Autodesk Inventor part; units mm, degrees
ref_plane "YZ Plane" through (0, 0, 0) normal (1, 0, 0) x (0, 1, 0)
ref_plane "XZ Plane" through (0, 0, 0) normal (0, 1, 0) x (-1, 0, 0)
ref_plane "XY Plane" through (0, 0, 0) normal (0, 0, 1) x (1, 0, 0)
ref_plane "Work Plane1" through (-71.5431, 15.4261, 39.8011) normal (1, 0, 0) x (0, -1, 0)
sketch "Sketch1" plane through (-71.5431, 15.4261, 39.8011) normal (1, 0, 0) x (0, -1, 0)
  circle A0 centre (-40.9, -21) radius 3
  circle A1 centre (-1.5, -21) radius 3
  line L0 (-45.9, -13) -> (3.5, -13)
  line L1 (3.5, -13) -> (3.5, -35)
  line L2 (3.5, -35) -> (-45.9, -35)
  line L3 (-45.9, -35) -> (-45.9, -13)
  line L4 (66.8457, -32) -> (-83.1543, -32)
  point P0 (15.4261, 39.8011)
  dimension "d0" = 5
  dimension "d1" = 8
  dimension "d2" = 5
  dimension "d3" = 3
extrude "Extrusion1" add sketch "Sketch1" along normal blind 12
sketch "Sketch2" plane through (-71.5431, 11.9261, 52.8011) normal (0, -1, 0) x (1, 0, 0)
  circle A0 centre (8.688, 16) radius 3
  circle A1 centre (8.688, 16) radius 3.75
  point P0 (71.5431, -52.8011)
  dimension "d6" = 7.5
extrude "Extrusion2" cut sketch "Sketch2" against normal through all contours A0 | A1
ref_plane "Work Plane2" through (-71.5431, 36.6261, 52.8011) normal (0, -1, 0) x (1, 0, 0)
sketch "Sketch3" plane through (-71.5431, 36.6261, 52.8011) normal (0, -1, 0) x (1, 0, 0)
  circle A0 centre (8.688, 16) radius 6
  circle A1 centre (8.688, 16) radius 6.5
  point P0 (71.5431, -52.8011)
  dimension "d9" = 0.5
extrude "Extrusion3" cut sketch "Sketch3" along normal mid plane 20 contours A0 | A1
sketch "Sketch5" plane through (-71.5431, 11.9261, 52.8011) normal (0, 0, -1) x (-1, 0, 0)
  circle A0 centre (-5.5, 42.2) radius 2.1
  arc A1 (-5.5, 5.1) -> (-5.5, 9.3) centre (-5.5, 7.2) ccw
  circle A2 centre (-5.5, 42.2) radius 1.45
  circle A3 centre (-5.5, 7.2) radius 1.45
  point P0 (-71.5431, -11.9261)
  dimension "d14" = 2.9
  dimension "d15" = 2.9
extrude "Extrusion5" cut sketch "Sketch5" against normal through all contours A2 | A3
properties part number "02_Opentrons_stage_x"
Work out the finished part from the listing and answer in its coordinate system (mm). A direction names the side the tool comes from. Round coordinates to 2 decimals unless told otherwise and drop trailing zeros. Loops run counter-clockwise (first coordinate to the right, second up) from the corner with the lowest first, then second, coordinate; pieces in that order, holes last. Notation, with made-up numbers: (3.25, 71) - (15.25, 71) arc R20 cw to (15.25, 84) - close; hole circle Ø9 at (5, 85). An arc over 180 degrees is marked (long way). One line per item, written item: value.
Q1. Find section D-D on y = 55. Give the vertices of the cut face in (x, z).
Check values:
outline: (-71.54, 52.8) - (-67.2, 52.8) - (-67.2, 58.11) - (-71.54, 58.11) - close; (-71.54, 63.49) - (-67.2, 63.49) - (-67.2, 74.8) - (-71.54, 74.8) - close; (-64.89, 52.8) - (-59.54, 52.8) - (-59.54, 58.11) - (-64.89, 58.11) - close; (-64.89, 63.49) - (-59.54, 63.49) - (-59.54, 67.04) arc R3.75 cw to (-64.89, 65.65) - close; (-64.89, 71.95) arc R3.75 cw to (-59.54, 70.56) - (-59.54, 74.8) - (-64.89, 74.8) - close
Q2. For faces 1 (the cylindrical face through (-64.41, 53.87, 65.39)), 2 (the flat face through (-67, 26.626, 69)), determine the directions among +Z, -Z, +X, -X, +Y, -Y from which every point of the face is accessible in a straight line to the end or side of a thin tool.
Check values:
face 1: +Y, -Y
face 2: none
Q3. Find section A-A on z = 61.5. Give the vertices of the cut face in (x, y).
Check values:
outline: (-71.54, 11.93) - (-59.54, 11.93) - (-59.54, 14.01) - (-71.54, 14.01) - close; (-71.54, 19.84) - (-67.3, 19.84) arc R1.45 cw to (-64.78, 19.84) - (-59.54, 19.84) - (-59.54, 53.41) - (-64.78, 53.41) arc R1.45 cw to (-67.3, 53.41) - (-71.54, 53.41) - close; (-71.54, 59.24) - (-59.54, 59.24) - (-59.54, 61.33) - (-71.54, 61.33) - close
Q4. Find section B-B on x = -61. Give the vertices of the cut face in (y, z), and give its area (3 significant figures).
Check values:
outline: (11.93, 52.8) - (61.33, 52.8) - (61.33, 65.54) - (46.63, 65.54) - (46.63, 62.57) - (26.63, 62.57) - (26.63, 65.54) - (11.93, 65.54) - close; (11.93, 72.06) - (26.63, 72.06) - (26.63, 74.8) - (11.93, 74.8) - close; (46.63, 72.06) - (61.33, 72.06) - (61.33, 74.8) - (46.63, 74.8) - close; hole circle Ø6 at (16.93, 60.8); hole circle Ø6 at (56.33, 60.8)
area: 594 mm2
Q5. Straight lines are drawn through the part: probe 1 along Y at (x, z) = (-64.25, 60.25); probe 2 along Y at (x, z) = (-67.25, 64.25); probe 3 along Y at (x, z) = (-66.5, 54). For each, find the intervals that lie inside material, in ascending order.
Check values:
probe 1: 11.93 to 13.98, 19.88 to 53.38, 59.28 to 61.33
probe 2: 11.93 to 18.32, 19.93 to 26.63, 46.63 to 53.32, 54.93 to 61.33
probe 3: 11.93 to 17.75, 20.5 to 52.75, 55.5 to 61.33
Q6. The mould has two halves that part along Z. Classify faces 3 (the flat face through (-67, 46.626, 69)), 4 (the flat face through (-66, 36, 74.801)), 5 (the flat face through (-59.543, 37, 60)): +Z half, -Z half, draft (parallel to the pull), parting line (faces both ways), or undercut.
Check values:
face 3: undercut
face 4: +Z half
face 5: draft
Q7. Find section C-C on y = 43.5. Give the vertices of the cut face in (x, z), and give its area (3 significant figures).
Check values:
outline: (-71.54, 52.8) - (-59.54, 52.8) - (-59.54, 63.21) arc R6.5 cw (long way) to (-65.36, 74.8) - (-71.54, 74.8) - close; (-60.36, 74.8) arc R6.5 cw to (-59.54, 74.39) - (-59.54, 74.8) - close
area: 158 mm2
